Part model, mm, in its own coordinate system. A direction names the side the tool comes from. Give positions to 0.01 mm unless a question says otherwise; leave off trailing zeros. Write each loop counter-clockwise with the first axis right and the second up, starting at its lowest first coordinate (ties: lowest second). Pieces come first, ordered by that corner, then holes. Notation, with made-up numbers: M 11.25,27.5 L 47.25,27.5 A30 cw 47.25,64.5 Z; hole C 9.25,-13.75 d5. An arc over 180 degrees is marked long. Use CSV: the item, a comma, the result in double quotes. Start each with the question number.
Item 1: Cut at A-A (x = 0). List the corners of the cut face in (y, z).
Item 2: Mould opens along Y. For faces 1 (the flat face through (-10, -6, 99)), 2 (the flat face through (4, 0, 99)), 3 (the flat face through (0, 4, 99)) say: released by +Y, released by -Y, zero draft, split by the parting line, or undercut.
Item 3: Which spindle directions (+Z, -Z, +X, -X, +Y, -Y) get a long thin tool onto all of the face, cutting with end or side? Do faces 4 (the flat face through (0, -4, 99)), 5 (the flat face through (10, 6, 99)). Say none if no direction does.
Item 4: Drill centre lines: line 1 (Y direction, x = 0, z = 154); line 2 (Y direction, x = 7.75, z = 50.5); line 3 (Y direction, x = 5, z = 185.5). Where is each one in solid material? Low to high. Write a range as [from, to].
Item 5: Pin check, flat tips, straight feed: pin 1 (1 mm diameter, centred on y = 9, z = 81, fed in from -X); pin 2 (3 mm diameter, centred on x = 1.5, z = 90.5, fed in from -Y); pin 3 (5 mm diameter, centred on y = 0.5, z = 136.5, fed in from +X). Stop position of each tip, or through.
from build123d import *

# Parameters (mm, degrees)
SKETCH_1_R      = 2.5
EXTRUDE_1_DEPTH = 200
FILLET_1_R      = 2


with BuildPart() as part:
    # 草图1 → 凸台-拉伸1 (new body)
    with BuildSketch(Plane.XY):
        Polygon((-3.151471863, 4), (3.151471863, 4), (5.45, 6.298528137), (5.45, 8.2), (3.1, 8.2), (3.1, 9.1), (3.6, 9.1), (3.6, 10), (10, 10), (10, 3.6), (9.1, 3.6), (9.1, 3.1), (8.2, 3.1), (8.2, 5.45), (6.298528137, 5.45), (4, 3.151471863), (4, -3.151471863), (6.298528137, -5.45), (8.2, -5.45), (8.2, -3.1), (9.1, -3.1), (9.1, -3.6), (10, -3.6), (10, -10), (3.6, -10), (3.6, -9.1), (3.1, -9.1), (3.1, -8.2), (5.45, -8.2), (5.45, -6.298528137), (3.151471863, -4), (-3.151471863, -4), (-5.45, -6.298528137), (-5.45, -8.2), (-3.1, -8.2), (-3.1, -9.1), (-3.6, -9.1), (-3.6, -10), (-10, -10), (-10, -3.6), (-9.1, -3.6), (-9.1, -3.1), (-8.2, -3.1), (-8.2, -5.45), (-6.298528137, -5.45), (-4, -3.151471863), (-4, 3.151471863), (-6.298528137, 5.45), (-8.2, 5.45), (-8.2, 3.1), (-9.1, 3.1), (-9.1, 3.6), (-10, 3.6), (-10, 10), (-3.6, 10), (-3.6, 9.1), (-3.1, 9.1), (-3.1, 8.2), (-5.45, 8.2), (-5.45, 6.298528137), align=None)
        Circle(SKETCH_1_R, mode=Mode.SUBTRACT)
    extrude(amount=EXTRUDE_1_DEPTH)

    # 圆角1
    fillet_1_edges = [part.edges().sort_by_distance(p)[0] for p in [
        (10, -10, 100),
        (-10, -10, 100),
        (-10, 10, 100),
        (10, 10, 100),
    ]]
    fillet(fillet_1_edges, radius=FILLET_1_R)


solid = part.part
Worked answers:
1,outline,"M -4,0 L -2.5,0 L -2.5,200 L -4,200 Z; M 2.5,0 L 4,0 L 4,200 L 2.5,200 Z"
2,face 1,"zero draft"
2,face 2,"undercut"
2,face 3,"released by +Y"
3,face 4,"+Z, -Z, -Y"
3,face 5,"+Z, -Z, +X, +Y, -Y"
4,line 1,"y = [-4, -2.5], [2.5, 4]"
4,line 2,"y = [-10, -5.45], [5.45, 10]"
4,line 3,"y = [-10, -8.2], [-5.85, -4.15], [4.15, 5.85], [8.2, 10]"
5,pin 1,"stops at x = -9.94"
5,pin 2,"stops at y = -4"
5,pin 3,"stops at x = 4"
